from build123d import *

# Parameters (mm, degrees)
SKETCH1_R           = 7.5565
SKETCH1_W           = 2.54
SKETCH1_H           = 4.572
BOSS_EXTRUDE1_DEPTH = 3.175


with BuildPart() as part:
    # Sketch1 → Boss-Extrude1 (new body)
    with BuildSketch(Plane.XY):
        with BuildLine():
            Line((-8.255, 15.639992312), (31.115, 15.639992312))
            ThreePointArc((31.115, 15.639992312), (35.156115254, 13.966107566), (36.83, 9.924992312))
            Line((36.83, 9.924992312), (36.83, -9.924992312))
            ThreePointArc((36.83, -9.924992312), (35.156115254, -13.966107566), (31.115, -15.639992312))
            Line((31.115, -15.639992312), (-8.255, -15.639992312))
            ThreePointArc((-8.255, -15.639992312), (-12.296115254, -13.966107566), (-13.97, -9.924992312))
            Line((-13.97, -9.924992312), (-13.97, 9.924992312))
            ThreePointArc((-13.97, 9.924992312), (-12.296115254, 13.966107566), (-8.255, 15.639992312))
        make_face()
        Circle(SKETCH1_R, mode=Mode.SUBTRACT)
        with Locations((22.86, 0)):
            Circle(SKETCH1_R, mode=Mode.SUBTRACT)
        with Locations((8.636, 12.083992312)):
            Rectangle(SKETCH1_W, SKETCH1_H, mode=Mode.SUBTRACT)
        with Locations((14.224, 12.083992312)):
            Rectangle(SKETCH1_W, SKETCH1_H, mode=Mode.SUBTRACT)
        with Locations((14.224, -12.083992312)):
            Rectangle(SKETCH1_W, SKETCH1_H, mode=Mode.SUBTRACT)
        with Locations((8.636, -12.083992312)):
            Rectangle(SKETCH1_W, SKETCH1_H, mode=Mode.SUBTRACT)
    extrude(amount=BOSS_EXTRUDE1_DEPTH)


solid = part.part
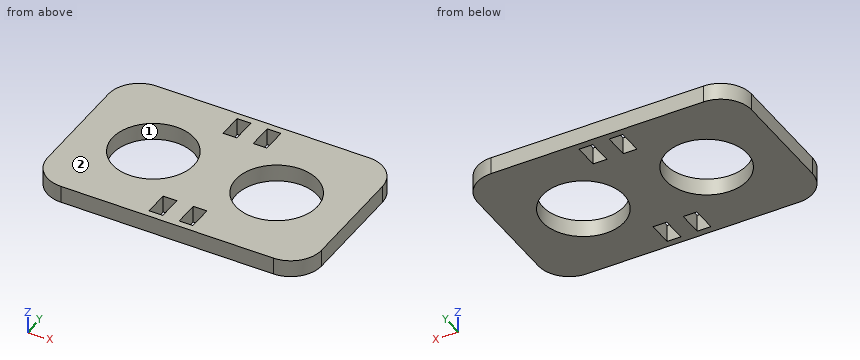
CAD build for the part. Positions are in the model's coordinates, mm. Face numbers are marked on the shaded views. Coordinates: 2 decimals unless noted, no trailing zeros. Loops run counter-clockwise (first coordinate to the right, second up) from the corner with the lowest first, then second, coordinate; pieces in that order, holes last. Notation, with made-up numbers: (35.25, 63.5) - (84.25, 63.5) arc R13 cw to (84.25, 73.5) - close; hole circle Ø8 at (-25, -3.5). An arc over 180 degrees is marked (long way). Write item = value, one per line. Start each with the question number.
Q1. Cut at A-A, the plane x = 22.86. List the corners of the cut face in (y, z) (1 decimal).
Q2. Cut at C-C, the plane z = 1.35. List the corners of the cut face in (x, y) (1 decimal), then the cut area to 3 significant figures.
Q3. Cut at D-D, the plane y = 12.5. List the corners of the cut face in (x, z) (3 decimals).
Q4. Flat gauge pins, fed straight in: pin 1 Ø1.6 at (y, z) = (-13, 1.5) entering from +X; pin 2 Ø13.5 at (x, y) = (22.86, 0) entering from -Z; pin 3 Ø1.6 at (y, z) = (12, 2) entering from +X; pin 4 Ø1 at (y, z) = (11, 1.5) entering from +X. Where does each tip first touch, or does it go through?
Q5. Drill centre lines: L1, parallel to Y at x = 0, z = 1.8; L2, parallel to X at y = -0.5, z = 2; L3, parallel to X at y = 14, z = 2.55. Where is each one in solid material? Low to high.
Q6. Pull direction Y, two halves, no side cores. Call the marked faces 1 and 2: pulls with the +Y half, pulls with the -Y half, needs draft (parallel to the pull), parting line crosses it, or undercut.
Q7. Cut at B-B, the plane y = 0. List the corners of the cut face in (x, z) (1 decimal), then the cut area to 3 significant figures.
Computed:
q1.outline = (-15.6, 0) - (-7.6, 0) - (-7.6, 3.2) - (-15.6, 3.2) - close; (7.6, 0) - (15.6, 0) - (15.6, 3.2) - (7.6, 3.2) - close
q2.outline = (-14, -9.9) arc R5.7 ccw to (-8.3, -15.6) - (31.1, -15.6) arc R5.7 ccw to (36.8, -9.9) - (36.8, 9.9) arc R5.7 ccw to (31.1, 15.6) - (-8.3, 15.6) arc R5.7 ccw to (-14, 9.9) - close; hole circle Ø15.1 at (0, 0); hole (7.4, -14.4) - (9.9, -14.4) - (9.9, -9.8) - (7.4, -9.8) - close; hole (7.4, 9.8) - (9.9, 9.8) - (9.9, 14.4) - (7.4, 14.4) - close; hole (13, -14.4) - (15.5, -14.4) - (15.5, -9.8) - (13, -9.8) - close; hole (13, 9.8) - (15.5, 9.8) - (15.5, 14.4) - (13, 14.4) - close; hole circle Ø15.1 at (22.9, 0)
q2.area = 1,160 mm²
q3.outline = (-13.357, 0) - (7.366, 0) - (7.366, 3.175) - (-13.357, 3.175) - close; (9.906, 0) - (12.954, 0) - (12.954, 3.175) - (9.906, 3.175) - close; (15.494, 0) - (36.217, 0) - (36.217, 3.175) - (15.494, 3.175) - close
q4.pin_1 = 36.36
q4.pin_2 = through
q4.pin_3 = 36.69
q4.pin_4 = 36.8
q5.L1 = -15.64 to -7.56, 7.56 to 15.64
q5.L2 = -13.97 to -7.54, 7.54 to 15.32, 30.4 to 36.83
q5.L3 = -12.26 to 7.37, 9.91 to 12.95, 15.49 to 35.12
q6.face_1 = undercut
q6.face_2 = needs draft
q7.outline = (-14, 0) - (-7.6, 0) - (-7.6, 3.2) - (-14, 3.2) - close; (7.6, 0) - (15.3, 0) - (15.3, 3.2) - (7.6, 3.2) - close; (30.4, 0) - (36.8, 0) - (36.8, 3.2) - (30.4, 3.2) - close
q7.area = 65.3 mm²
